The model under review builds one solid part; all positions refer to its coordinate system, in mm. A direction names the side the tool comes from. Round coordinates to 2 decimals unless told otherwise and drop trailing zeros. Order: outer loops, then holes, each group sorted by start corner. A loop starts at its lowest first (then second) coordinate and runs counter-clockwise, first axis right, second up. Notation, with made-up numbers: M 51,-8.75 L 74,-8.75 A20 ccw 74,23.25 Z; hole C -2,-25 d5. An arc over 180 degrees is marked long. Use a Markdown table: item, result. Add a question column.
1. For faces 4 (the cylindrical face through (9.03, 6.27, 1.68)), 5 (the cylindrical face through (-0.7, -11, 1.6)), list the 3-axis set-ups (+Z, -Z, +X, -X, +Y, -Y) from which the entire face can be reached by the end or side of a thin tool; tool diameter is ignored.
2. The part is to be moulded in two halves that separate along Y. For faces 1 (the cylindrical face through (3.441, 15.497, 3.757)), 2 (the cylindrical face through (6.869, 9.724, 4.126)), 3 (the flat face through (-7, 0, 7.62)), say which applies: +Y half, -Y half, draft (parallel to the pull), parting line (faces both ways), or undercut.
3. Consider section A-A on x = 0. State the section outline as (y, z) points (3 decimals).
4. To check wall thickness, follow probe 1 along X at (y, z) = (5.5, 2.5); probe 2 along X at (y, z) = (1, 2.75); probe 3 along X at (y, z) = (-11.5, 5.75). State the ranges of each line that lie inside material, in increasing order.
5. Consider section B-B on z = 5.25. Count the separate pieces of the cut face and the enclosed holes in it, then the cut area to 3 significant figures.
6. Insertion check: P1, Ø3, axis at y = -3, z = 1, coming from the -X side; P2, Ø4, axis at y = -9, z = 6.5, coming from the -X side; P3, Ø4, axis at x = 10.5, z = 1.5, coming from the +Y side. Each pin has a flat end and moves straight along its axis. Give the tip position at first contact, or say it passes through.
7. Consider section C-C on y = -3. State the section outline as (x, z) points.
from build123d import *

# Parameters (mm, degrees)
SKETCH1_R                                = 15.875
BOSS_EXTRUDE1_DEPTH                      = 7.62
SKETCH2_R                                = 6.35
CUT_EXTRUDE1_DEPTH                       = 24.708556472
CIRPATTERN1_COUNT                        = 3
F_1_16_0_0625_DIAMETER_HOLE1_D           = 1.5875
F_1_16_0_0625_DIAMETER_HOLE1_CSINK_D     = 2.8575
F_1_16_0_0625_DIAMETER_HOLE1_CSINK_ANGLE = 100
CIRPATTERN2_COUNT                        = 2


with BuildPart() as part:
    # Sketch1 → Boss-Extrude1 (new body)
    with BuildSketch(Plane.XY):
        with Locations(Location((0, 0, 0), (0, 0, 180))):
            Circle(SKETCH1_R)
    extrude(amount=BOSS_EXTRUDE1_DEPTH)

    # Sketch2 → Cut-Extrude1 (cut, through all)
    with BuildSketch(Plane.XY.offset(7.62)):
        Circle(SKETCH2_R)
    extrude(amount=-CUT_EXTRUDE1_DEPTH, mode=Mode.SUBTRACT)

    # Sketch36 → 3/16 (0.1875) Diameter Hole1 (revolve, cut)
    with BuildSketch(Plane(origin=(0, -15.875, 3.877224023), x_dir=(0, 0, -1), z_dir=(1, 0, 0))):
        Polygon((0, 0), (0, 20.480799349), (2.38125, 19.05), (2.38125, 0), align=None)
    f_3_16_0_1875_diameter_hole1 = revolve(axis=Axis((0, -22.225, 3.877224023), (0, 1, 0)), mode=Mode.SUBTRACT)

    # CirPattern1: 3/16 (0.1875) Diameter Hole1 ×3 about axis
    cirpattern1_axis = Axis((0, 0, 7.62), (0, 0, -1))
    for i in range(1, CIRPATTERN1_COUNT):
        add(f_3_16_0_1875_diameter_hole1.rotate(cirpattern1_axis, i * 360 / CIRPATTERN1_COUNT), mode=Mode.SUBTRACT)

    # 1/16 (0.0625) Diameter Hole1 (through all)
    with Locations(Plane(origin=(0, 0, 0), x_dir=(-1, 0, 0), z_dir=(0, 0, -1))):
        with Locations((-6.442291542, 9.054531238)):
            f_1_16_0_0625_diameter_hole1 = CounterSinkHole(F_1_16_0_0625_DIAMETER_HOLE1_D / 2, F_1_16_0_0625_DIAMETER_HOLE1_CSINK_D / 2, counter_sink_angle=F_1_16_0_0625_DIAMETER_HOLE1_CSINK_ANGLE)

    # CirPattern2: 1/16 (0.0625) Diameter Hole1 ×2 about axis
    cirpattern2_axis = Axis((0, 0, 0), (0, 0, 1))
    for i in range(1, CIRPATTERN2_COUNT):
        add(f_1_16_0_0625_diameter_hole1.rotate(cirpattern2_axis, i * 360 / CIRPATTERN2_COUNT), mode=Mode.SUBTRACT)


solid = part.part
Answer block:
| question | item | result |
|---|---|---|
| 1 | face 4 | none |
| 1 | face 5 | -Y |
| 2 | face 1 | parting line |
| 2 | face 2 | undercut |
| 2 | face 3 | draft |
| 3 | outline | M -15.875,0 L -6.35,0 L -6.35,1.496 L -15.875,1.496 Z; M -15.875,6.258 L -6.35,6.258 L -6.35,7.62 L -15.875,7.62 Z; M 6.35,0 L 15.875,0 L 15.875,7.62 L 6.35,7.62 Z |
| 4 | probe 1 | -14.89 to -13.41, -5.64 to -3.17, 3.17 to 5.64, 13.41 to 14.89 |
| 4 | probe 2 | -15.84 to -6.27, 6.27 to 15.84 |
| 4 | probe 3 | -10.94 to -1.47, 1.47 to 10.94 |
| 5 | separate pieces | 3 |
| 5 | enclosed holes | 2 |
| 5 | area | 549 mm^2 |
| 6 | P1 | x = -15.8 |
| 6 | P2 | x = -14.25 |
| 6 | P3 | y = 13.41 |
| 7 | outline | M -15.59,0 L -5.6,0 L -5.6,7.62 L -15.59,7.62 Z; M 5.6,0 L 15.59,0 L 15.59,7.62 L 5.6,7.62 Z |
